```python
from build123d import *

# Parameters (mm, degrees)
SKETCH1_W           = 116.54028
SKETCH1_H           = 101.7397
SKETCH1_R           = 1.6002
BOSS_EXTRUDE1_DEPTH = 1.65608
SKETCH2_W           = 11.69924
SKETCH2_H           = 11.99896
BOSS_EXTRUDE2_DEPTH = 4.5
SKETCH3_R           = 3.5
BOSS_EXTRUDE3_DEPTH = 7
CHAMFER1_SIZE       = 0.5
SKETCH5_R           = 3
BOSS_EXTRUDE4_DEPTH = 8


with BuildPart() as part:
    # Sketch1 → Boss-Extrude1 (new body)
    with BuildSketch(Plane.XY):
        Rectangle(SKETCH1_W, SKETCH1_H)
        with Locations((-51.2699, 46.45025)):
            Circle(SKETCH1_R, mode=Mode.SUBTRACT)
        with Locations((50.76952, 46.45025)):
            Circle(SKETCH1_R, mode=Mode.SUBTRACT)
        with Locations((50.76952, -8.44931)):
            Circle(SKETCH1_R, mode=Mode.SUBTRACT)
        with Locations((-51.2699, -8.44931)):
            Circle(SKETCH1_R, mode=Mode.SUBTRACT)
    extrude(amount=BOSS_EXTRUDE1_DEPTH)

    # Sketch2 → Boss-Extrude2 (add)
    with BuildSketch(Plane.XY.offset(1.65608)):
        with Locations((-44.26966, -36.86937)):
            Rectangle(SKETCH2_W, SKETCH2_H)
        with Locations((44.26966, -36.86937)):
            Rectangle(SKETCH2_W, SKETCH2_H)
    extrude(amount=BOSS_EXTRUDE2_DEPTH)

    # Sketch3 → Boss-Extrude3 (add)
    with BuildSketch(Plane.XY.offset(6.15608)):
        with Locations((-44.26966, -36.86937)):
            Circle(SKETCH3_R)
        with Locations((44.26966, -36.86937)):
            Circle(SKETCH3_R)
    extrude(amount=BOSS_EXTRUDE3_DEPTH)

    # Chamfer1
    chamfer1_edges = [part.edges().sort_by_distance(p)[0] for p in [
        (-47.76966, -36.86937, 13.15608),
        (40.76966, -36.86937, 13.15608),
    ]]
    chamfer(chamfer1_edges, length=CHAMFER1_SIZE)

    # Sketch5 → Boss-Extrude4 (add)
    with BuildSketch(Plane.XY.offset(13.15608)):
        with Locations((44.26966, -36.86937)):
            Circle(SKETCH5_R)
        with Locations((-44.26966, -36.86937)):
            Circle(SKETCH5_R)
    extrude(amount=BOSS_EXTRUDE4_DEPTH)


solid = part.part
```
For this review, take the finished solid that the model builds, in its own axes (mm). A direction names the side the tool comes from. Give positions to 0.01 mm unless a question says otherwise; leave off trailing zeros. Write each loop counter-clockwise with the first axis right and the second up, starting at its lowest first coordinate (ties: lowest second). Pieces come first, ordered by that corner, then holes.
Item 1: Take a section at C-C (x = 8.5). Give the boundary of the cut face in (y, z), and give its area (3 significant figures).
Item 2: Take a section at B-B (y = 21.5). Give the boundary of the cut face in (x, z), and give its area (3 significant figures).
Item 3: Wall thickness on probe 1 along Z at (x, y) = (-46.5, 38); probe 2 along Y at (x, z) = (46, 5.5): over which ranges is each line inside the solid? List them lowest first.
Item 4: Take a section at D-D (z = 14.5). Give the boundary of the cut face in (x, y).
Item 5: Machinability: for faces 1 (the face through (-50.119, -37, 4)), 2 (the face through (-52.54, 45.48, 0.82)), 3 (the face through (-44, -42.869, 4)), 4 (the face through (-38.42, -37, 4)), 5 (the face through (-44.73, -33.4, 9.36)), which of the approach directions +Z, -Z, +X, -X, +Y, -Y give a long, thin tool a straight path to every point of the face, cutting with its end or side? Answer none if there is none.
Item 6: Insertion check: P1, Ø3.5, axis at y = -39, z = 5, coming from the -X side; P2, Ø1.3, axis at x = -45, z = 3, coming from the -Y side; P3, Ø12, axis at x = -1, y = -16.5, coming from the +Z side; P4, Ø4, axis at x = -51.27, y = -8.45, coming from the -Z side. Each pin has a flat end and moves straight along its axis. Give the tip position at first contact, or say it passes through.
Item 7: Take a section at A-A (z = 4). Give the boundary of the cut face in (x, y).
Item 8: The part is to be moulded in two halves that separate along Z. For faces 6 (the face through (44, -30.87, 4)), 7 (the face through (-42, -34, 6.156)), 8 (the face through (-1, 1, 0)), say which applies: +Z half, -Z half, draft (parallel to the pull), parting line (faces both ways), or undercut.
Established:
1. outline: (-50.87, 0) - (50.87, 0) - (50.87, 1.66) - (-50.87, 1.66) - close
1. area: 168 mm2
2. outline: (-58.27, 0) - (58.27, 0) - (58.27, 1.66) - (-58.27, 1.66) - close
2. area: 193 mm2
3. probe 1: z = 0 to 1.66
3. probe 2: y = -42.87 to -30.87
4. outline: circle Ø6 at (-44.27, -36.87); circle Ø6 at (44.27, -36.87)
5. face 1: +Z, -X, +Y, -Y
5. face 2: +Z, -Z
5. face 3: +Z, +X, -X, -Y
5. face 4: +Z, +Y, -Y
5. face 5: +Z
6. P1: stops at x = -50.12
6. P2: stops at y = -42.87
6. P3: stops at z = 1.66
6. P4: stops at z = 0
7. outline: (-50.12, -42.87) - (-38.42, -42.87) - (-38.42, -30.87) - (-50.12, -30.87) - close; (38.42, -42.87) - (50.12, -42.87) - (50.12, -30.87) - (38.42, -30.87) - close
8. face 6: draft
8. face 7: +Z half
8. face 8: -Z half
